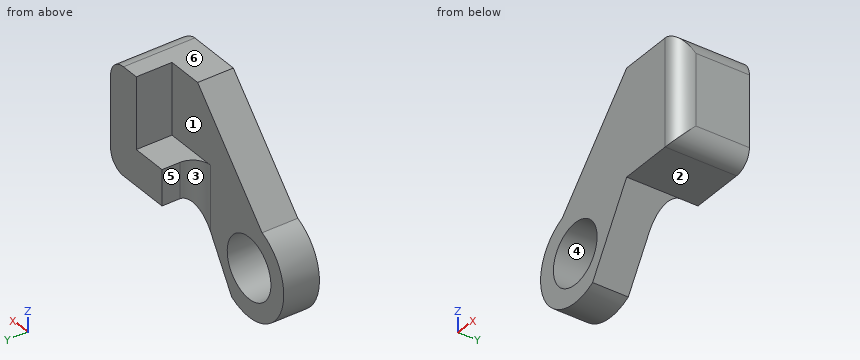
```python
from build123d import *

# Parameters (mm, degrees)
SKETCH1_W           = 20
SKETCH1_H           = 30
BOSS_EXTRUDE1_DEPTH = 10
BOSS_EXTRUDE2_DEPTH = 10
SKETCH4_R           = 8.5
BOSS_EXTRUDE3_DEPTH = 10
FILLET1_R           = 5


with BuildPart() as part:
    # Sketch1 → Boss-Extrude1 (new body)
    with BuildSketch(Plane(origin=(0, 0, 0), x_dir=(1, 0, 0), z_dir=(0, 1, 0))):
        with Locations((10, -15)):
            Rectangle(SKETCH1_W, SKETCH1_H)
    extrude(amount=BOSS_EXTRUDE1_DEPTH)

    # Sketch2 → Boss-Extrude2 (add)
    with BuildSketch(Plane(origin=(0, 10, 0), x_dir=(1, 0, 0), z_dir=(0, 1, 0))):
        Polygon((0, 0), (0, -10), (10, -10), (10, -30), (20, -30), (20, 0), align=None)
    extrude(amount=BOSS_EXTRUDE2_DEPTH)

    # Sketch4 → Boss-Extrude3 (add)
    with BuildSketch(Plane(origin=(0, 10, 0), x_dir=(1, 0, 0), z_dir=(0, 1, 0))):
        with BuildLine():
            Line((0, 0), (-13.247067503, 21.689649383))
            ThreePointArc((-13.247067503, 21.689649383), (-32.129444614, 15.92676753), (-25.072116083, -2.510940749))
            Line((-25.072116083, -2.510940749), (0, -30))
            Line((0, -30), (0, 0))
        make_face()
        with Locations(Location((-20, 10, 0), (0, 0, 270))):
            Circle(SKETCH4_R, mode=Mode.SUBTRACT)
    extrude(amount=-BOSS_EXTRUDE3_DEPTH)

    # Fillet1
    fillet1_edges = [part.edges().sort_by_distance(p)[0] for p in [
        (0, 10, 5),
        (20, 0, 15),
        (20, 10, 0),
        (20, 10, 30),
    ]]
    fillet(fillet1_edges, radius=FILLET1_R)


solid = part.part
```
The model under review builds one solid part; all positions refer to its coordinate system, in mm. Face numbers are marked on the shaded views. A direction names the side the tool comes from. Round coordinates to 2 decimals unless told otherwise and drop trailing zeros. Write each loop counter-clockwise with the first axis right and the second up, starting at its lowest first coordinate (ties: lowest second). Pieces come first, ordered by that corner, then holes. Notation, with made-up numbers: (80.25, 11) - (115.25, 11) arc R19 ccw to (115.25, 25) - close; hole circle Ø10 at (52, 20). An arc over 180 degrees is marked (long way). Use one line per item in the form item = value.
Q1. Tool access review of the marked faces 1, 2 and 3: name each direction out of +Z, -Z, +X, -X, +Y, -Y from which nothing blocks a thin tool from reaching the whole face with its end or side.
Answer key:
face_1 = +Z, -X, +Y
face_2 = -Z, +X, +Y, -Y
face_3 = +Z, -Z, -X, +Y
Q2. Draft analysis for pull direction X (two halves, no side actions). For the marked faces 4, 5 and 6, state which applies: +X half, -X half, draft (parallel to the pull), parting line (faces both ways), or undercut.
Answer key:
face_4 = undercut
face_5 = -X half
face_6 = draft
Q3. For line 1 (X direction, y = 17.75, z = 6); line 2 (X direction, y = 8, z = -10); line 3 (Y direction, x = -13.5, z = -20), list the stretches that pass through material, from the lowest coordinate up. Write a range as [from, to].
Answer key:
line_1 = [0, 20]
line_2 = [-33.5, -28.5], [-11.5, -6.11]
line_3 = [0, 10]
Q4. Insertion check: pin 1 Ø1 at (y, z) = (15.5, 19.5) entering from -X; pin 2 Ø12 at (x, y) = (11, 8) entering from -Z; pin 3 Ø8 at (y, z) = (13, 18.5) entering from -X. Each pin has a flat end and moves straight along its axis. Give the tip position at first contact, or say it passes through.
Answer key:
pin_1 = 10
pin_2 = 0
pin_3 = -12.9
Q5. Consider section D-D (y = 13.25). State the section outline as (x, z) points.
Answer key:
outline = (-0.32, -0.52) - (0, 0) - (15, 0) arc R5 ccw to (20, 5) - (20, 25) arc R5 ccw to (15, 30) - (10, 30) - (10, 10) - (-0.32, 10) - close
Q6. Consider section C-C (x = -27). State the section outline as (y, z) points, and give its area (3 significant figures).
Answer key:
outline = (0, -21.54) - (10, -21.54) - (10, -14.82) - (0, -14.82) - close; (0, -5.18) - (10, -5.18) - (10, 1.54) - (0, 1.54) - close
area = 134 mm2
Q7. Consider section B-B (z = -10). State the section outline as (x, y) points, and give its area (3 significant figures).
Answer key:
outline = (-33.5, 0) - (-28.5, 0) - (-28.5, 10) - (-33.5, 10) - close; (-11.5, 0) - (-6.11, 0) - (-6.11, 10) - (-11.5, 10) - close
area = 104 mm2
Q8. Consider section A-A (y = 7.5). State the section outline as (x, z) points, and give its area (3 significant figures).
Answer key:
outline = (-25.07, 2.51) arc R13.5 ccw (long way) to (-13.25, -21.69) - (0, 0) - (15, 0) arc R5 ccw to (20, 5) - (20, 25) arc R5 ccw to (15, 30) - (0, 30) - close; hole circle Ø17 at (-20, -10)
area = 1,340 mm2
